CAD build for the part. Positions are in the model's coordinates, mm. Face numbers are marked on the shaded views. A direction names the side the tool comes from. Coordinates: 2 decimals unless noted, no trailing zeros. Write each loop counter-clockwise with the first axis right and the second up, starting at its lowest first coordinate (ties: lowest second). Pieces come first, ordered by that corner, then holes. Notation, with made-up numbers: (15.25, -24) -> (36.25, -24) arc R22 cw to (36.25, 15) -> close; hole circle Ø9 at (58.5, -8.75). An arc over 180 degrees is marked (long way). Answer as CSV lines item,"result".
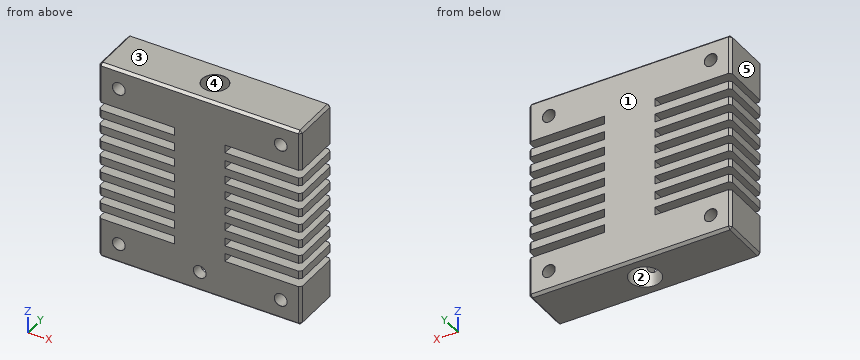
```python
from build123d import *

# Parameters (mm, degrees)
ESQUISSE1_W                                         = 40
ESQUISSE1_H                                         = 40
BOSS_EXTRU_1_DEPTH                                  = 10
DIAM_TRE_DU_PER_AGE_4_0_4_1_D                       = 4
TROU_POUR_TARAUDAGE_POUR_TROU_TARAUD_M6_D           = 5
TROU_POUR_TARAUDAGE_POUR_TROU_TARAUD_M6_DEPTH       = 8
TROU_POUR_TARAUDAGE_POUR_TROU_TARAUD_M6_CSINK_D     = 5.05
TROU_POUR_TARAUDAGE_POUR_TROU_TARAUD_M6_CSINK_ANGLE = 90
TROU_POUR_TARAUDAGE_POUR_TROU_TARAUD_M6_TIP         = 1.502151548
DIAM_TRE_DU_PER_AGE_6_0_6_1_D                       = 6
DIAM_TRE_DU_PER_AGE_6_0_6_1_DEPTH                   = 20
DIAM_TRE_DU_PER_AGE_6_0_6_1_TIP                     = 1.802581857
TROU_POUR_TARAUDAGE_POUR_TROU_TARAUD_2_COUNT        = 2
TROU_POUR_TARAUDAGE_POUR_TROU_TARAUD_2_PITCH        = 32
TROU_POUR_TARAUDAGE_POUR_TROU_TARAUD_3_COUNT        = 2
TROU_POUR_TARAUDAGE_POUR_TROU_TARAUD_3_PITCH        = 45.254833996
TROU_POUR_TARAUDAGE_POUR_TROU_TARAUD_4_COUNT        = 2
TROU_POUR_TARAUDAGE_POUR_TROU_TARAUD_4_PITCH        = 32
TROU_POUR_TARAUDAGE_POUR_TROU_TARAUD_5_D            = 2.5
TROU_POUR_TARAUDAGE_POUR_TROU_TARAUD_5_DEPTH        = 5
TROU_POUR_TARAUDAGE_POUR_TROU_TARAUD_5_CSINK_D      = 2.55
TROU_POUR_TARAUDAGE_POUR_TROU_TARAUD_5_CSINK_ANGLE  = 90
TROU_POUR_TARAUDAGE_POUR_TROU_TARAUD_5_TIP          = 0.751075774
ESQUISSE21_W                                        = 15
ESQUISSE21_H                                        = 1.6
ENL_V_MAT_EXTRU_1_DEPTH                             = 58.445626535
R_P_TITION_LIN_AIRE1_COUNT                          = 8
R_P_TITION_LIN_AIRE1_PITCH                          = 3.2
CHANFREIN1_SIZE                                     = 0.5


with BuildPart() as part:
    # Esquisse1 → Boss.-Extru.1 (new body)
    with BuildSketch(Plane(origin=(0, 0, 0), x_dir=(1, 0, 0), z_dir=(0, 1, 0))):
        with Locations((20, 20)):
            Rectangle(ESQUISSE1_W, ESQUISSE1_H)
    extrude(amount=BOSS_EXTRU_1_DEPTH)

    # Diamètre du perçage Ø4.0 (4)1 (through all)
    with Locations(Plane.XY):
        with Locations((20, 5)):
            Hole(DIAM_TRE_DU_PER_AGE_4_0_4_1_D / 2)

    # Trou pour taraudage pour trou taraudé M61
    with Locations(Plane.XY):
        with Locations((20, 5)):
            CounterSinkHole(TROU_POUR_TARAUDAGE_POUR_TROU_TARAUD_M6_D / 2, TROU_POUR_TARAUDAGE_POUR_TROU_TARAUD_M6_CSINK_D / 2, depth=TROU_POUR_TARAUDAGE_POUR_TROU_TARAUD_M6_DEPTH, counter_sink_angle=TROU_POUR_TARAUDAGE_POUR_TROU_TARAUD_M6_CSINK_ANGLE)
            with Locations((0, 0, -(TROU_POUR_TARAUDAGE_POUR_TROU_TARAUD_M6_DEPTH + TROU_POUR_TARAUDAGE_POUR_TROU_TARAUD_M6_TIP / 2))):  # 118° drill point
                Cone(0, TROU_POUR_TARAUDAGE_POUR_TROU_TARAUD_M6_D / 2, TROU_POUR_TARAUDAGE_POUR_TROU_TARAUD_M6_TIP, mode=Mode.SUBTRACT)

    # Diamètre du perçage Ø6.0 (6)1
    with Locations(Plane(origin=(0, 0, -40), x_dir=(-1, 0, 0), z_dir=(0, 0, -1))):
        with Locations((-20, 5)):
            Hole(DIAM_TRE_DU_PER_AGE_6_0_6_1_D / 2, depth=DIAM_TRE_DU_PER_AGE_6_0_6_1_DEPTH)
            with Locations((0, 0, -(DIAM_TRE_DU_PER_AGE_6_0_6_1_DEPTH + DIAM_TRE_DU_PER_AGE_6_0_6_1_TIP / 2))):  # 118° drill point
                Cone(0, DIAM_TRE_DU_PER_AGE_6_0_6_1_D / 2, DIAM_TRE_DU_PER_AGE_6_0_6_1_TIP, mode=Mode.SUBTRACT)

    # Esquisse17 → Trou pour taraudage pour trou taraud_ M3 (revolve, cut)
    with BuildSketch(Plane(origin=(4, 0, -4), x_dir=(0, 0, -1), z_dir=(1, 0, 0))):
        Polygon((0, 0), (0, 10), (1.275, 10), (1.25, 9.975), (1.25, 0.025), (1.275, 0), align=None)
    trou_pour_taraudage_pour_trou_taraud_m3 = revolve(axis=Axis((4, -6.35, -4), (0, 1, 0)), mode=Mode.SUBTRACT)

    # Trou pour taraudage pour trou taraud 2: Trou pour taraudage pour trou taraud_ M3 ×2
    with Locations(*[(i * TROU_POUR_TARAUDAGE_POUR_TROU_TARAUD_2_PITCH, 0, 0) for i in range(1, TROU_POUR_TARAUDAGE_POUR_TROU_TARAUD_2_COUNT)]):
        add(trou_pour_taraudage_pour_trou_taraud_m3, mode=Mode.SUBTRACT)

    # Trou pour taraudage pour trou taraud 3: Trou pour taraudage pour trou taraud_ M3 ×2
    with Locations(*[Vector(0.7071067811865475, 0, -0.7071067811865476) * (i * TROU_POUR_TARAUDAGE_POUR_TROU_TARAUD_3_PITCH) for i in range(1, TROU_POUR_TARAUDAGE_POUR_TROU_TARAUD_3_COUNT)]):
        add(trou_pour_taraudage_pour_trou_taraud_m3, mode=Mode.SUBTRACT)

    # Trou pour taraudage pour trou taraud 4: Trou pour taraudage pour trou taraud_ M3 ×2
    with Locations(*[(0, 0, -i * TROU_POUR_TARAUDAGE_POUR_TROU_TARAUD_4_PITCH) for i in range(1, TROU_POUR_TARAUDAGE_POUR_TROU_TARAUD_4_COUNT)]):
        add(trou_pour_taraudage_pour_trou_taraud_m3, mode=Mode.SUBTRACT)

    # Trou pour taraudage pour trou taraud 5
    with Locations(Plane(origin=(0, 0, 0), x_dir=(-1, 0, 0), z_dir=(0, -1, 0))):
        with Locations((-20, 36)):
            CounterSinkHole(TROU_POUR_TARAUDAGE_POUR_TROU_TARAUD_5_D / 2, TROU_POUR_TARAUDAGE_POUR_TROU_TARAUD_5_CSINK_D / 2, depth=TROU_POUR_TARAUDAGE_POUR_TROU_TARAUD_5_DEPTH, counter_sink_angle=TROU_POUR_TARAUDAGE_POUR_TROU_TARAUD_5_CSINK_ANGLE)
            with Locations((0, 0, -(TROU_POUR_TARAUDAGE_POUR_TROU_TARAUD_5_DEPTH + TROU_POUR_TARAUDAGE_POUR_TROU_TARAUD_5_TIP / 2))):  # 118° drill point
                Cone(0, TROU_POUR_TARAUDAGE_POUR_TROU_TARAUD_5_D / 2, TROU_POUR_TARAUDAGE_POUR_TROU_TARAUD_5_TIP, mode=Mode.SUBTRACT)

    # Esquisse21 → Enlèv. mat.-Extru.1 (cut, through all)
    with BuildSketch(Plane.XZ):
        with Locations((7.5, -8.8)):
            Rectangle(ESQUISSE21_W, ESQUISSE21_H)
        with Locations((32.5, -8.8)):
            Rectangle(ESQUISSE21_W, ESQUISSE21_H)
    enl_v_mat_extru_1 = extrude(amount=-ENL_V_MAT_EXTRU_1_DEPTH, mode=Mode.SUBTRACT)

    # Répétition linéaire1: Enlèv. mat.-Extru.1 ×8
    with Locations(*[(0, 0, -i * R_P_TITION_LIN_AIRE1_PITCH) for i in range(1, R_P_TITION_LIN_AIRE1_COUNT)]):
        add(enl_v_mat_extru_1, mode=Mode.SUBTRACT)

    # Chanfrein1
    chanfrein1_edges = [part.edges().sort_by_distance(p)[0] for p in [
        (40, 10, -4),
        (0, 0, -10.4),
        (0, 10, -10.4),
        (40, 0, -13.6),
        (40, 10, -13.6),
        (20, 10, -40),
        (0, 0, -13.6),
        (0, 10, -13.6),
        (40, 0, -16.8),
        (40, 10, -16.8),
        (0, 0, -16.8),
        (0, 10, -16.8),
        (40, 0, -20),
        (40, 10, -20),
        (0, 0, -20),
        (0, 10, -20),
        (40, 0, -23.2),
        (40, 10, -23.2),
        (0, 0, -23.2),
        (0, 10, -23.2),
        (40, 0, -26.4),
        (40, 10, -26.4),
        (0, 0, -26.4),
        (0, 10, -26.4),
        (40, 0, -29.6),
        (40, 10, -29.6),
        (0, 0, -29.6),
        (0, 10, -29.6),
        (40, 0, -36),
        (40, 10, -36),
        (0, 10, -36),
        (20, 0, -40),
        (40, 0, -4),
        (20, 0, 0),
        (0, 0, -36),
        (20, 10, 0),
        (0, 0, -4),
        (0, 5, -40),
        (40, 5, -40),
        (0, 10, -4),
        (40, 5, 0),
        (0, 5, 0),
        (40, 0, -10.4),
        (40, 10, -10.4),
    ]]
    chamfer(chanfrein1_edges, length=CHANFREIN1_SIZE)


solid = part.part
```
Item 1: Saw through at A-A on z = -36. State how many separate pieces and enclosed holes the cut face has, and give its area (3 significant figures).
Answer below:
separate pieces,"3"
enclosed holes,"0"
area,"316 mm2"
Item 2: Flat gauge pins, fed straight in: pin 1 (2 mm diameter, centred on x = 36, z = -36, fed in from +Y); pin 2 (0.5 mm diameter, centred on y = 5.5, z = -18.5, fed in from -X). Where does each tip first touch, or does it go through?
Answer below:
pin 1,"passes through"
pin 2,"stops at x = 15"
Item 3: Two-plate mould, pull along Y, no slides. Class the marked faces 1, 2 and 3: pulls with the +Y half, pulls with the -Y half, needs draft (parallel to the pull), parting line crosses it, or undercut.
Answer below:
face 1,"pulls with the +Y half"
face 2,"undercut"
face 3,"needs draft"
Item 4: Saw through at D-D on z = -25. Give the cut face in (x, y).
Answer below:
outline,"(15, 0) -> (25, 0) -> (25, 10) -> (15, 10) -> close; hole circle Ø6 at (20, 5)"
Item 5: Wall check: line 1 (X direction, y = 5.75, z = -4); line 2 (X direction, y = 7.25, z = -5); line 3 (X direction, y = 5, z = -27.5). Give the ranges that are in metal, low to high. Write a range as from..to.
Answer below:
line 1,"x = 0..2.75, 5.25..17.62, 22.38..34.75, 37.25..40"
line 2,"x = 0..3.25, 4.75..18.91, 21.09..35.25, 36.75..40"
line 3,"x = 15..17, 23..25"
Item 6: 3-axis set-ups, long thin cutter, end or side, ignore diameter. For the marked faces 4 and 5: which of +Z, -Z, +X, -X, +Y, -Y reach the whole face in a straight line?
Answer below:
face 4,"+Z"
face 5,"+Z, -Z, -X, +Y, -Y"
Item 7: Saw through at B-B on x = 20. Give the cut face in (y, z) (3 decimals), and give its area (3 significant figures).
Answer below:
outline,"(0, -39.5) -> (0.5, -40) -> (2, -40) -> (2, -37.25) -> (0.025, -37.25) -> (0, -37.275) -> close; (0, -34.725) -> (0.025, -34.75) -> (2, -34.75) -> (2, -20) -> (3, -19.399) -> (3, -8.3) -> (2.5, -8) -> (2.5, -0.025) -> (2.475, 0) -> (0.5, 0) -> (0, -0.5) -> close; (7, -19.399) -> (8, -20) -> (8, -40) -> (9.5, -40) -> (10, -39.5) -> (10, -0.5) -> (9.5, 0) -> (7.525, 0) -> (7.5, -0.025) -> (7.5, -8) -> (7, -8.3) -> close"
area,"186 mm2"
